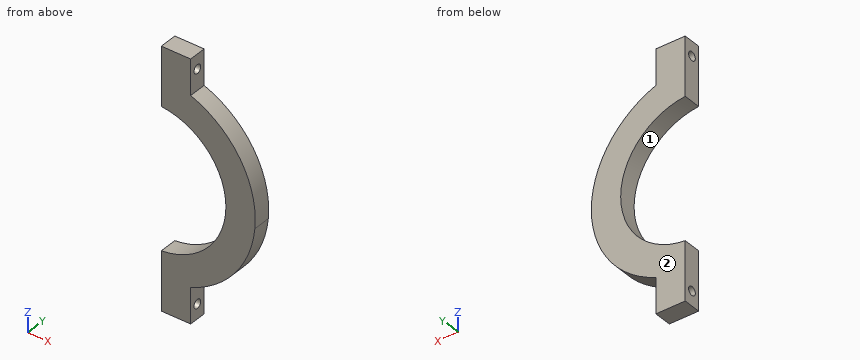
```python
from build123d import *

# Parameters (mm, degrees)
BOSS_EXTRUDE1_DEPTH = 6
SKETCH4_R           = 1.5
CUT_EXTRUDE3_DEPTH  = 11


with BuildPart() as part:
    # Sketch1 → Boss-Extrude1 (new body)
    with BuildSketch(Plane(origin=(0, 0, 0), x_dir=(1, 0, 0), z_dir=(0, 1, 0))):
        with BuildLine():
            Line((2, 43.916521486), (2, 23.916521486))
            ThreePointArc((2, 23.916521486), (24, 0), (2, -23.916521486))
            Line((2, -23.916521486), (2, -43.916521486))
            Line((2, -43.916521486), (12, -43.916521486))
            Line((12, -43.916521486), (12, -31.811947441))
            ThreePointArc((12, -31.811947441), (28.791009913, -18.085290934), (33.867388444, 3))
            ThreePointArc((33.867388444, 3), (27.082954224, 20.55513538), (12, 31.811947441))
            Line((12, 31.811947441), (12, 43.916521486))
            Line((12, 43.916521486), (2, 43.916521486))
        make_face()
    extrude(amount=BOSS_EXTRUDE1_DEPTH)

    # Sketch4 → Cut-Extrude3 (cut, through all)
    with BuildSketch(Plane(origin=(12, 0, 0), x_dir=(0, 0, -1), z_dir=(1, 0, 0))):
        with Locations((-38.916521486, 3)):
            Circle(SKETCH4_R)
    cut_extrude3 = extrude(amount=-CUT_EXTRUDE3_DEPTH, mode=Mode.SUBTRACT)

    # Mirror1: Cut-Extrude3 across plane
    add(cut_extrude3.mirror(Plane.XY), mode=Mode.SUBTRACT)


solid = part.part
```
Design review of the part built by this model. Coordinates are the model's own, in mm. Face numbers are marked on the shaded views. Coordinates: 2 decimals unless noted, no trailing zeros. Loops run counter-clockwise (first coordinate to the right, second up) from the corner with the lowest first, then second, coordinate; pieces in that order, holes last. Notation, with made-up numbers: M -1,-7 L 11,-7 A25 ccw 11,22 Z; hole C -2,63.25 d3. An arc over 180 degrees is marked long. One line per question, with ' | ' between items.
(1) We need section D-D (z = -26.5). Give the boundary of the cut face in (x, y).
Filled in:
outline: M 2,0 L 21.3,0 L 21.3,6 L 2,6 Z
(2) We need section A-A (y = 3). Give the boundary of the cut face in (x, z), and give its area (3 significant figures).
Filled in:
outline: M 2,-43.92 L 12,-43.92 L 12,-40.42 L 2,-40.42 Z; M 2,-37.42 L 12,-37.42 L 12,-31.81 A34 ccw 12,31.81 L 12,37.42 L 2,37.42 L 2,23.92 A24 cw 2,-23.92 Z; M 2,40.42 L 12,40.42 L 12,43.92 L 2,43.92 Z | area: 1,030 mm^2
(3) Wall thickness on probe 1 along Z at (x, y) = (11.5, 1.85); probe 2 along X at (y, z) = (0.6, 32); probe 3 along Z at (x, y) = (22, 3.5): over which ranges is each line inside the solid? List them lowest first.
Filled in:
probe 1: z = -43.92 to -39.88, -37.95 to -21.07, 21.07 to 37.95, 39.88 to 43.92 | probe 2: x = 2 to 12 | probe 3: z = -25.92 to -9.59, 9.59 to 25.92
(4) Draft analysis for pull direction Z (two halves, no side actions). For the marked faces 1 and 2, state which applies: released by +Z, released by -Z, zero draft, split by the parting line, or undercut.
Filled in:
face 1: undercut | face 2: zero draft
(5) We need section B-B (x = 20). Give the boundary of the cut face in (y, z).
Filled in:
outline: M 0,-27.5 L 6,-27.5 L 6,-13.27 L 0,-13.27 Z; M 0,13.27 L 6,13.27 L 6,27.5 L 0,27.5 Z
(6) We need section C-C (x = 7). Give the boundary of the cut face in (y, z).
Filled in:
outline: M 0,-43.92 L 6,-43.92 L 6,-22.96 L 0,-22.96 Z; M 0,22.96 L 6,22.96 L 6,43.92 L 0,43.92 Z; hole C 3,-38.92 d3; hole C 3,38.92 d3
(7) For pin 1 Ø8 at (x, z) = (30.5, -24.5) entering from +Y; pin 2 Ø3 at (y, z) = (4.5, -38.5) entering from +X, all flat-tipped, find the tip position at first contact; note any pin that passes through.
Filled in:
pin 1: passes through | pin 2: stops at x = 12
